Study the drawing (mm; zero at the part's minimum x, y, z) and answer. A direction names the side the tool comes from. Give positions to 0.01 mm unless a question says otherwise; leave off trailing zeros. Write each loop counter-clockwise with the first axis right and the second up, starting at its lowest first coordinate (ties: lowest second). Pieces come first, ordered by that corner, then holes. Notation, with made-up numbers: (71.25, 45.25) - (75.25, 45.25) arc R21 cw to (75.25, 66.25) - close; hole circle Ø2 at (-23, 39). An arc over 180 degrees is marked (long way). Answer as CSV lines item,"result".
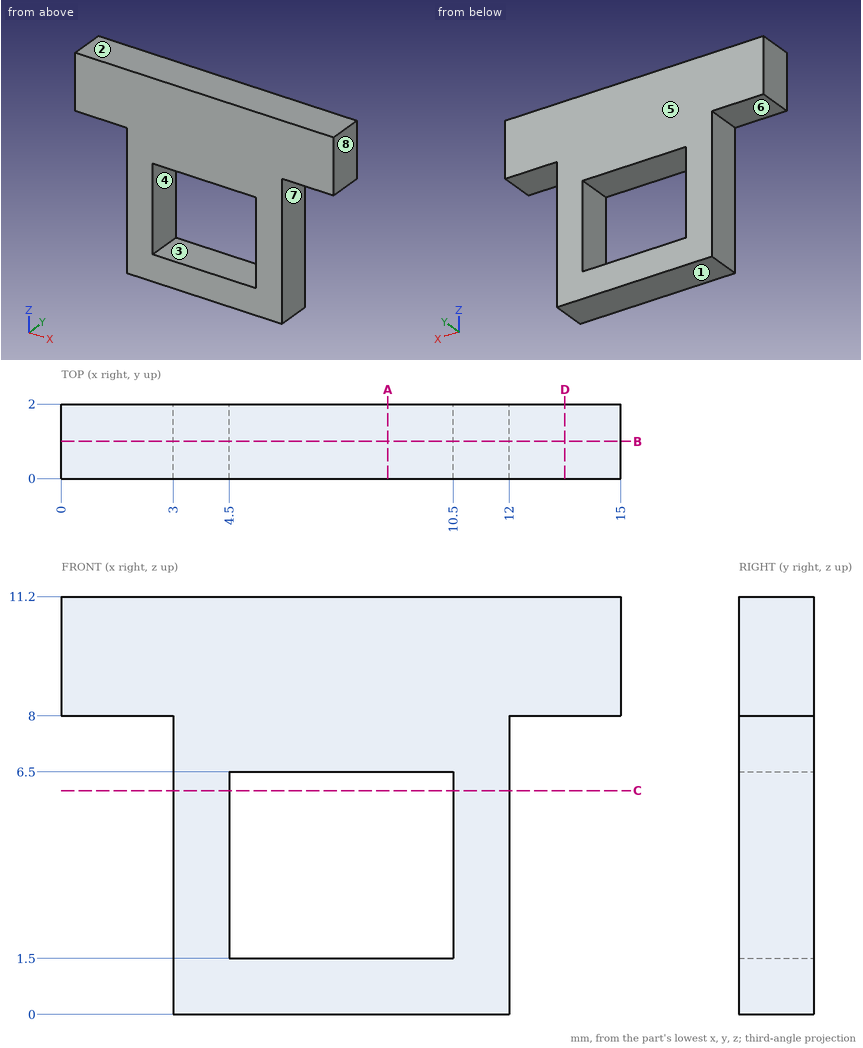
(1) For the marked faces 4, 5, 6, 7 and 8, determine the directions among +Z, -Z, +X, -X, +Y, -Y from which every point of the face is accessible in a straight line to the end or side of a thin tool.
Worked out:
face 4,"+Y, -Y"
face 5,"+Z, -Z, +X, -X, +Y"
face 6,"-Z, -X, +Y, -Y"
face 7,"-Z, +X, +Y, -Y"
face 8,"+Z, -Z, +X, +Y, -Y"
(2) A cutting plane is placed at D-D (x = 13.5). Write down the section's boundary in (y, z).
Worked out:
outline,"(0, 8) - (2, 8) - (2, 11.2) - (0, 11.2) - close"
(3) Find the intervals of material crossed by L1, parallel to X at y = 0.2, z = 6.25; L2, parallel to Z at x = 7.5, y = 0.7; L3, parallel to X at y = 1.5, z = 7.75, in increasing order.
Worked out:
L1,"x = 3 to 4.5, 10.5 to 12"
L2,"z = 0 to 1.5, 6.5 to 11.2"
L3,"x = 3 to 12"
(4) Each of these flat-tipped pins is pushed along its axis until it touches: P1, Ø1, axis at x = 2, y = 1, coming from the -Z side; P2, Ø0.6, axis at y = 1, z = 3, coming from the +X side. Where does it stop, or does it pass through?
Worked out:
P1,"stops at z = 8"
P2,"stops at x = 12"
(5) A cutting plane is placed at B-B (y = 1). Write down the section's boundary in (x, z), and give its area (3 significant figures).
Worked out:
outline,"(0, 8) - (3, 8) - (3, 0) - (12, 0) - (12, 8) - (15, 8) - (15, 11.2) - (0, 11.2) - close; hole (4.5, 1.5) - (10.5, 1.5) - (10.5, 6.5) - (4.5, 6.5) - close"
area,"90.0 mm^2"
(6) A cutting plane is placed at A-A (x = 8.75). Write down the section's boundary in (y, z), and give its area (3 significant figures).
Worked out:
outline,"(0, 0) - (2, 0) - (2, 1.5) - (0, 1.5) - close; (0, 6.5) - (2, 6.5) - (2, 11.2) - (0, 11.2) - close"
area,"12.4 mm^2"
(7) A cutting plane is placed at C-C (z = 6). Write down the section's boundary in (x, y).
Worked out:
outline,"(3, 0) - (4.5, 0) - (4.5, 2) - (3, 2) - close; (10.5, 0) - (12, 0) - (12, 2) - (10.5, 2) - close"
(8) The mould has two halves that part along Z. Classify the marked faces 1, 2 and 3: +Z half, -Z half, draft (parallel to the pull), parting line (faces both ways), or undercut.
Worked out:
face 1,"-Z half"
face 2,"+Z half"
face 3,"undercut"
